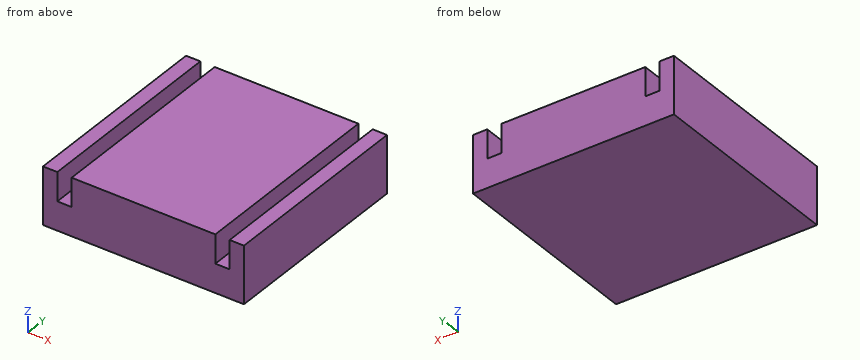
```python
from build123d import *

# Parameters (mm, degrees)
F0_W     = 5
F0_H     = 70
F1_DEPTH = 20
F0_W_2   = 50.2
F0_W_3   = 2.5
F2_DEPTH = 10


with BuildPart() as f1:
    # F0 (on Top) → F1 (new body)
    with BuildSketch(Plane.XY):
        with Locations((-53.9031001925, 1.7255722731)):
            Rectangle(F0_W, F0_H)
    extrude(amount=F1_DEPTH)



with BuildPart() as f1b:
    # F0 (on Top) → F1, piece 2 (new body)
    with BuildSketch(Plane.XY):
        with Locations((-21.3031001925, 1.7255722731)):
            Rectangle(F0_W_2, F0_H)
    extrude(amount=F1_DEPTH)


with BuildPart() as f1c:
    # F0 (on Top) → F1, piece 3 (new body)
    with BuildSketch(Plane.XY):
        with Locations((11.2968998075, 1.7255722731)):
            Rectangle(F0_W, F0_H)
    extrude(amount=F1_DEPTH)


with BuildPart() as f1_1:
    add(f1.part)

    add(f1b.part)  # F2 merges F1b

    add(f1c.part)  # F2 merges F1c
    # F0 (on Top) → F2 (join)
    with BuildSketch(Plane.XY):
        with Locations((-47.6531001925, 1.7255722731)):
            Rectangle(F0_W_3, F0_H)
        with Locations((-50.1531001925, 1.7255722731)):
            Rectangle(F0_W_3, F0_H)
        with Locations((5.0468998075, 1.7255722731)):
            Rectangle(F0_W_3, F0_H)
        with Locations((7.5468998075, 1.7255722731)):
            Rectangle(F0_W_3, F0_H)
    extrude(amount=F2_DEPTH)


solid = f1_1.part
```
The listing builds one solid part. Answer for the finished solid, in the listing's coordinates (mm). Coordinates: 2 decimals unless noted, no trailing zeros. Order: outer loops, then holes, each group sorted by start corner. A loop starts at its lowest first (then second) coordinate and runs counter-clockwise, first axis right, second up. Notation, with made-up numbers: M -31.5,35 L 7.5,35 A22 ccw 7.5,61 Z; hole C 84,87 d5. An arc over 180 degrees is marked long. Answer as a JSON object with one key per item and string values. Group by question number.
1. Flat-ended cylindrical pins translate along their axes: P1, Ø1.5, axis at x = 6, y = 12, coming from the +Z side; P2, Ø1, axis at x = -9, y = 28.5, coming from the -Z side. Find the tip coordinate at first contact, or state that the pin passes through.
2. Straight lines are drawn through the part: line 1 (X direction, y = 1, z = 13.5); line 2 (Z direction, x = -48.5, y = 29). For each, find the intervals that lie inside material, in ascending order.
3. Section A-A on z = 11.25 is taken. Write down the section's boundary in (x, y).
4. Section B-B on y = -5 is taken. Write down the section's boundary in (x, z), then the cut area to 3 significant figures.
5. Section C-C on x = 7.5 is taken. Write down the section's boundary in (y, z).
Values follow:
{
 "1": {"P1": "z = 10", "P2": "z = 0"},
 "2": {"line 1": "-56.4 to -51.4, -46.4 to 3.8, 8.8 to 13.8", "line 2": "0 to 10"},
 "3": {"outline": "M -56.4,-33.27 L -51.4,-33.27 L -51.4,36.73 L -56.4,36.73 Z; M -46.4,-33.27 L 3.8,-33.27 L 3.8,36.73 L -46.4,36.73 Z; M 8.8,-33.27 L 13.8,-33.27 L 13.8,36.73 L 8.8,36.73 Z"},
 "4": {"outline": "M -56.4,0 L 13.8,0 L 13.8,20 L 8.8,20 L 8.8,10 L 3.8,10 L 3.8,20 L -46.4,20 L -46.4,10 L -51.4,10 L -51.4,20 L -56.4,20 Z", "area": "1,300 mm2"},
 "5": {"outline": "M -33.27,0 L 36.73,0 L 36.73,10 L -33.27,10 Z"}
}
